Geometry check sheet. Reference: the model listing, model coordinates, mm. Round coordinates to 2 decimals unless told otherwise and drop trailing zeros. Write each loop counter-clockwise with the first axis right and the second up, starting at its lowest first coordinate (ties: lowest second). Pieces come first, ordered by that corner, then holes. Notation, with made-up numbers: M 43.25,87 L 88.25,87 A32 cw 88.25,115 Z; hole C 89.25,10.25 d2. An arc over 180 degrees is marked long. Use a Markdown table: item, result.
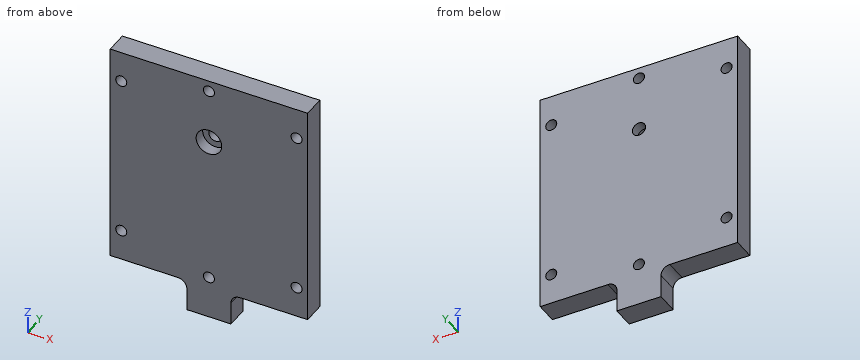
```python
from build123d import *

# Parameters (mm, degrees)
ESQUISSE1_R             = 1.5
EXTRUSION1_DEPTH        = 5
TROU_TARAUD_M3X0_51_D   = 2.5
ESQUISSE6_R             = 2.9
ENL_V_MAT_EXTRU_3_DEPTH = 49.536712909


with BuildPart() as part:
    # Esquisse1 → Extrusion1 (new body)
    with BuildSketch(Plane(origin=(0, 0, 0), x_dir=(1, 0, 0), z_dir=(0, 1, 0))):
        with BuildLine():
            Line((-22.35, 35.8), (-7, 35.8))
            ThreePointArc((-7, 35.8), (-5.585786438, 36.385786438), (-5, 37.8))
            Line((-5, 37.8), (-5, 43))
            Line((-5, 43), (5, 43))
            Line((5, 43), (5, 37.8))
            ThreePointArc((5, 37.8), (5.585786438, 36.385786438), (7, 35.8))
            Line((7, 35.8), (22.35, 35.8))
            Line((22.35, 35.8), (22.35, -15))
            Line((22.35, -15), (-22.35, -15))
            Line((-22.35, -15), (-22.35, 35.8))
        make_face()
        with Locations(Location((0, 0, 0), (0, 0, 270))):
            Circle(ESQUISSE1_R, mode=Mode.SUBTRACT)
    extrude(amount=EXTRUSION1_DEPTH)

    # Trou taraud_ M3x0.51 (through all)
    with Locations(Plane(origin=(0, 5, 0), x_dir=(-1, 0, 0), z_dir=(0, 1, 0))):
        with Locations((0, -33.3), (-19.85, -28.8), (-19.85, 8), (0, 12.5), (19.85, -28.8), (19.85, 8)):
            Hole(TROU_TARAUD_M3X0_51_D / 2)

    # Esquisse6 → Enl_v. mat.-Extru.3 (cut, through all)
    with BuildSketch(Plane(origin=(0, 2.7, 0), x_dir=(1, 0, 0), z_dir=(0, 1, 0))):
        with Locations(Location((0, 0, 0), (0, 0, 270))):
            Circle(ESQUISSE6_R)
    extrude(amount=-ENL_V_MAT_EXTRU_3_DEPTH, mode=Mode.SUBTRACT)


solid = part.part
```
Item 1: Cross-section at B-B, the plane x = 0. Record the cut outline in (y, z).
Outcome:
| item | result |
|---|---|
| outline | M 0,-43 L 5,-43 L 5,-34.55 L 0,-34.55 Z; M 0,-32.05 L 5,-32.05 L 5,-1.5 L 2.7,-1.5 L 2.7,-2.9 L 0,-2.9 Z; M 0,2.9 L 2.7,2.9 L 2.7,1.5 L 5,1.5 L 5,11.25 L 0,11.25 Z; M 0,13.75 L 5,13.75 L 5,15 L 0,15 Z |
Item 2: Material ranges on line 1 along Z through (x, y) = (-20, 0.4); line 2 along X through (y, z) = (3.7, 0); line 3 along Z through (x, y) = (0, 3.5), recorded low to high. Write a range as from..to.
Outcome:
| item | result |
|---|---|
| line 1 | z = -35.8..-30.04, -27.56..6.76, 9.24..15 |
| line 2 | x = -22.35..-1.5, 1.5..22.35 |
| line 3 | z = -43..-34.55, -32.05..-1.5, 1.5..11.25, 13.75..15 |
Item 3: Cross-section at C-C, the plane y = 3.8. Record the cut outline in (x, z), and give its area (3 significant figures).
Outcome:
| item | result |
|---|---|
| outline | M -22.35,-35.8 L -7,-35.8 A2 cw -5,-37.8 L -5,-43 L 5,-43 L 5,-37.8 A2 cw 7,-35.8 L 22.35,-35.8 L 22.35,15 L -22.35,15 Z; hole C -19.85,-28.8 d2.5; hole C -19.85,8 d2.5; hole C 0,0 d3; hole C 0,-33.3 d2.5; hole C 0,12.5 d2.5; hole C 19.85,-28.8 d2.5; hole C 19.85,8 d2.5 |
| area | 2,310 mm2 |
Item 4: Cross-section at D-D, the plane x = 19.85. Record the cut outline in (y, z).
Outcome:
| item | result |
|---|---|
| outline | M 0,-35.8 L 5,-35.8 L 5,-30.05 L 0,-30.05 Z; M 0,-27.55 L 5,-27.55 L 5,6.75 L 0,6.75 Z; M 0,9.25 L 5,9.25 L 5,15 L 0,15 Z |
Item 5: Cross-section at A-A, the plane z = -33.3. Record the cut outline in (x, y), and give its area (3 significant figures).
Outcome:
| item | result |
|---|---|
| outline | M -22.35,0 L -1.25,0 L -1.25,5 L -22.35,5 Z; M 1.25,0 L 22.35,0 L 22.35,5 L 1.25,5 Z |
| area | 211 mm2 |
Item 6: Go/stop test with flat-tipped pins: pin 1 (9.5 mm diameter, centred on x = 0, z = 0, fed in from -Y); pin 2 (1.5 mm diameter, centred on x = -11.5, y = 1.5, fed in from -Z); pin 3 (1.7 mm diameter, centred on x = 1, z = 0.5, fed in from -Y). Record where each tip stops, or that it passes through.
Outcome:
| item | result |
|---|---|
| pin 1 | stops at y = 0 |
| pin 2 | stops at z = -35.8 |
| pin 3 | stops at y = 2.7 |
